```python
from build123d import *

# Parameters (mm, degrees)
SKETCH1_R           = 3.429
SKETCH1_R_2         = 2.54
BOSS_EXTRUDE1_DEPTH = 3.2004
SKETCH2_R           = 2.159
CUT_EXTRUDE1_DEPTH  = 3.2004
SKETCH5_R           = 1.7272
SKETCH5_W           = 40.894
SKETCH5_H           = 20.32
CUT_EXTRUDE3_DEPTH  = 4.2004
CUT_EXTRUDE4_DEPTH  = 3.2004
CUT_EXTRUDE8_DEPTH  = 3.2004
SKETCH11_W          = 107.95
SKETCH11_H          = 3.2512
CUT_EXTRUDE9_DEPTH  = 3.2004
SKETCH12_R          = 2.2479
CUT_EXTRUDE10_DEPTH = 3.2004
BOSS_EXTRUDE2_DEPTH = 3.2004


with BuildPart() as part:
    # Sketch1 → Boss-Extrude1 (new body)
    with BuildSketch(Plane.XY):
        with BuildLine():
            Line((0, 0), (120.015, 0))
            ThreePointArc((120.015, 0), (130.351788397, 3.075697789), (137.325636158, 11.302152593))
            Line((137.325636158, 11.302152593), (155.257499999, 52.11572))
            ThreePointArc((155.257499999, 52.11572), (157.462147967, 67.664529981), (151.26869294, 82.095991421))
            ThreePointArc((151.26869294, 82.095991421), (55.081013593, 128.103082212), (-41.106665754, 82.095991421))
            ThreePointArc((-41.106665754, 82.095991421), (-46.904819593, 67.459968464), (-43.385473773, 52.11572))
            Line((-43.385473773, 52.11572), (-19.648099871, 11.302152593))
            ThreePointArc((-19.648099871, 11.302152593), (-11.333429333, 3.027112684), (0, 0))
        make_face()
        with Locations((120.015, 18.90776)):
            Circle(SKETCH1_R, mode=Mode.SUBTRACT)
        with Locations((0, 18.90776)):
            Circle(SKETCH1_R_2, mode=Mode.SUBTRACT)
        with Locations((19.734727626, 25.566426992)):
            Circle(SKETCH1_R_2, mode=Mode.SUBTRACT)
        with Locations((99.400822531, 30.809360911)):
            Circle(SKETCH1_R_2, mode=Mode.SUBTRACT)
    extrude(amount=BOSS_EXTRUDE1_DEPTH)

    # Sketch2 → Cut-Extrude1 (cut)
    with BuildSketch(Plane(origin=(0, 0, 0), x_dir=(-1, 0, 0), z_dir=(0, 0, -1))):
        with Locations((-92.0115, 52.115719911)):
            Circle(SKETCH2_R)
        with Locations((-28.0035, 52.115719911)):
            Circle(SKETCH2_R)
        with Locations((-98.1075, 3.81)):
            Circle(SKETCH2_R)
        with Locations((-21.9075, 3.81)):
            Circle(SKETCH2_R)
    extrude(amount=-CUT_EXTRUDE1_DEPTH, mode=Mode.SUBTRACT)

    # Sketch5 → Cut-Extrude3 (cut, through all)
    with BuildSketch(Plane(origin=(0, 0, 0), x_dir=(-1, 0, 0), z_dir=(0, 0, -1))):
        with Locations((-98.932021292, 23.90776)):
            Circle(SKETCH5_R)
        with Locations((-48.432021292, 13.90776)):
            Circle(SKETCH5_R)
        with Locations((-48.432021292, 23.90776)):
            Circle(SKETCH5_R)
        with Locations((-98.932021292, 13.90776)):
            Circle(SKETCH5_R)
        with Locations((-73.682021292, 18.90776)):
            Rectangle(SKETCH5_W, SKETCH5_H)
    extrude(amount=-CUT_EXTRUDE3_DEPTH, mode=Mode.SUBTRACT)

    # Sketch6 → Cut-Extrude4 (cut)
    with BuildSketch(Plane.XY.offset(3.2004)):
        with BuildLine():
            Line((49.171021292, 19.92376), (53.235021292, 19.92376))
            Line((53.235021292, 19.92376), (53.235021292, 17.89176))
            Line((53.235021292, 17.89176), (49.171021292, 17.89176))
            ThreePointArc((49.171021292, 17.89176), (48.155021292, 18.90776), (49.171021292, 19.92376))
        make_face()
        with BuildLine():
            Line((94.129021292, 19.92376), (98.193021292, 19.92376))
            ThreePointArc((98.193021292, 19.92376), (99.209021292, 18.90776), (98.193021292, 17.89176))
            Line((98.193021292, 17.89176), (94.129021292, 17.89176))
            Line((94.129021292, 17.89176), (94.129021292, 19.92376))
        make_face()
    extrude(amount=-CUT_EXTRUDE4_DEPTH, mode=Mode.SUBTRACT)

    # Sketch10 → Cut-Extrude8 (cut)
    with BuildSketch(Plane(origin=(0, 0, 0), x_dir=(-1, 0, 0), z_dir=(0, 0, -1))):
        with BuildLine():
            Line((-34.3535, 78.785719911), (-21.6535, 78.785719911))
            ThreePointArc((-21.6535, 78.785719911), (-18.4785, 75.610719911), (-21.6535, 72.435719911))
            Line((-21.6535, 72.435719911), (-34.3535, 72.435719911))
            ThreePointArc((-34.3535, 72.435719911), (-37.5285, 75.610719911), (-34.3535, 78.785719911))
        make_face()
    extrude(amount=-CUT_EXTRUDE8_DEPTH, mode=Mode.SUBTRACT)

    # Sketch11 → Cut-Extrude9 (cut)
    with BuildSketch(Plane(origin=(0, 0, 0), x_dir=(-1, 0, 0), z_dir=(0, 0, -1))):
        with Locations((-60.0075, 46.680119911)):
            Rectangle(SKETCH11_W, SKETCH11_H)
    extrude(amount=-CUT_EXTRUDE9_DEPTH, mode=Mode.SUBTRACT)

    # Sketch12 → Cut-Extrude10 (cut)
    with BuildSketch(Plane(origin=(0, 0, 0), x_dir=(-1, 0, 0), z_dir=(0, 0, -1))):
        with Locations((-142.479014632, 18.224067698)):
            Circle(SKETCH12_R)
        with Locations((3.91433865, 18.224067698)):
            Circle(SKETCH12_R)
    extrude(amount=-CUT_EXTRUDE10_DEPTH, mode=Mode.SUBTRACT)

    # Sketch13 → Boss-Extrude2 (add)
    with BuildSketch(Plane(origin=(0, 0, 0), x_dir=(-1, 0, 0), z_dir=(0, 0, -1))):
        with BuildLine():
            Line((-83.804619012, 124.717903232), (20.105573885, 102.592791936))
            ThreePointArc((20.105573885, 102.592791936), (13.448555565, 111.243555983), (11.985080528, 122.060665224))
            ThreePointArc((11.985080528, 122.060665224), (-2.230930753, 150.611793246), (-34.052645197, 148.457639581))
            ThreePointArc((-34.052645197, 148.457639581), (-57.67418009, 133.958784174), (-83.804619012, 124.717903232))
        make_face()
    extrude(amount=-BOSS_EXTRUDE2_DEPTH)


solid = part.part
```
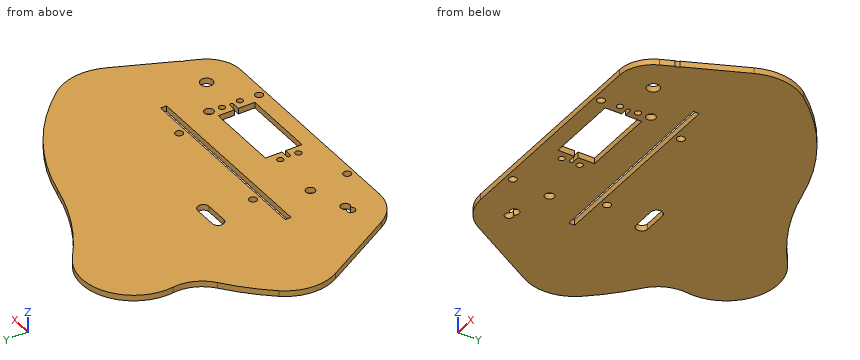
Geometry check sheet. Reference: the model listing, model coordinates, mm. Round coordinates to 2 decimals unless told otherwise and drop trailing zeros. Loops run counter-clockwise (first coordinate to the right, second up) from the corner with the lowest first, then second, coordinate; pieces in that order, holes last. Notation, with made-up numbers: (73, 30.25) - (80, 30.25) arc R18 ccw to (80, 62.25) - close; hole circle Ø3 at (54.5, 60.5). An arc over 180 degrees is marked (long way). Use a Markdown table: item, result.
Q1. Cross-section at C-C on z = 2.6. State how many separate pieces and enclosed holes the cut face has, plus the area to 3 significant figures.
Solutions:
| item | result |
|---|---|
| separate pieces | 1 |
| enclosed holes | 15 |
| area | 21,400 mm2 |
Q2. Go/stop test with a flat-tipped pin: P1, Ø1, axis at y = 22.5, z = 1, coming from the -X side. Record where the tip stops, or that it passes through.
Solutions:
| item | result |
|---|---|
| P1 | stops at x = -26.45 |
Q3. Cross-section at A-A on x = 106. Record the cut outline in (y, z), plus the area to 3 significant figures.
Solutions:
| item | result |
|---|---|
| outline | (0, 0) - (45.05, 0) - (45.05, 3.2) - (0, 3.2) - close; (48.31, 0) - (117.12, 0) - (117.12, 3.2) - (48.31, 3.2) - close |
| area | 364 mm2 |
Q4. Cross-section at D-D on y = 119.5. Record the cut outline in (x, z).
Solutions:
| item | result |
|---|---|
| outline | (-11.82, 0) - (100.38, 0) - (100.38, 3.2) - (-11.82, 3.2) - close |
Q5. Cross-section at B-B on y = 3.81. Record the cut outline in (x, z), plus the area to 3 significant figures.
Solutions:
| item | result |
|---|---|
| outline | (-12.6, 0) - (19.75, 0) - (19.75, 3.2) - (-12.6, 3.2) - close; (24.07, 0) - (95.95, 0) - (95.95, 3.2) - (24.07, 3.2) - close; (100.27, 0) - (131.4, 0) - (131.4, 3.2) - (100.27, 3.2) - close |
| area | 433 mm2 |
Q6. Material ranges on line 1 (Y direction, x = 64, z = 1.8); line 2 (X direction, y = 51.5, z = 1.1); line 3 (Y direction, x = 75, z = 2.4), recorded low to high.
Solutions:
| item | result |
|---|---|
| line 1 | y = 0 to 8.75, 29.07 to 45.05, 48.31 to 131.14 |
| line 2 | x = -43.03 to 25.93, 30.07 to 89.94, 94.08 to 154.99 |
| line 3 | y = 0 to 8.75, 29.07 to 45.05, 48.31 to 127.15 |
